```python
from build123d import *

# Parameters (mm, degrees)
BOSS_EXTRUDE1_DEPTH = 0.6


with BuildPart() as part:
    # Sketch1 → Boss-Extrude1 (new body)
    with BuildSketch(Plane(origin=(0, 0, 0), x_dir=(1, 0, 0), z_dir=(0, 1, 0))):
        with BuildLine():
            ThreePointArc((7.5, 10), (0, 12.5), (-7.5, 10))
            Line((-7.5, 10), (-7.5, 0.704545455))
            Line((-7.5, 0.704545455), (7.5, 0.704545455))
            Line((7.5, 0.704545455), (7.5, 10))
        make_face()
        with BuildLine():
            Line((-7.5, 0.704545455), (-7.5, 10))
            ThreePointArc((-7.5, 10), (-5.590169944, -11.180339887), (12.5, 0))
            ThreePointArc((12.5, 0), (11.180339887, 5.590169944), (7.5, 10))
            Line((7.5, 10), (7.5, 0.704545455))
            Line((7.5, 0.704545455), (-7.5, 0.704545455))
        make_face()
        with BuildLine():
            Line((7.5, 24.295454545), (-7.5, 24.295454545))
            Line((-7.5, 24.295454545), (-7.5, 10))
            ThreePointArc((-7.5, 10), (0, 12.5), (7.5, 10))
            Line((7.5, 10), (7.5, 24.295454545))
        make_face()
    extrude(amount=BOSS_EXTRUDE1_DEPTH)


solid = part.part
```
Check sheet for the modelled part. Datum: model origin and axes. Units: mm. Round coordinates to 2 decimals unless told otherwise and drop trailing zeros. Write each loop counter-clockwise with the first axis right and the second up, starting at its lowest first coordinate (ties: lowest second). Pieces come first, ordered by that corner, then holes. Notation, with made-up numbers: (-25, 8) -> (-14, 8) arc R28 ccw to (-14, 30) -> close; hole circle Ø3 at (56.5, -18). An arc over 180 degrees is marked (long way). One line per question, with ' | ' between items. Start each with the question number.
1. Sectioned sample at A-A, the plane y = 0.4. Record the cut outline in (x, z).
2. Scan lines: line 1 along X through (y, z) = (0.5, -13); line 2 along X through (y, z) = (0.45, -9.5); line 3 along Z through (x, y) = (-8.25, 0.3). Record each from-to range of solid material in increasing order. Write a range as from..to.
3. Sectioned sample at B-B, the plane z = 10. Record the cut outline in (x, y).
4. Sectioned sample at C-C, the plane x = 8.75. Record the cut outline in (y, z), then the cut area to 3 significant figures.
Taken from the geometry:
1) outline: (-7.5, -24.3) -> (7.5, -24.3) -> (7.5, -10) arc R12.5 ccw (long way) to (-7.5, -10) -> close
2) line 1: x = -7.5..7.5 | line 2: x = -8.12..8.12 | line 3: z = -9.39..9.39
3) outline: (-7.5, 0) -> (7.5, 0) -> (7.5, 0.6) -> (-7.5, 0.6) -> close
4) outline: (0, -8.93) -> (0.6, -8.93) -> (0.6, 8.93) -> (0, 8.93) -> close | area: 10.7 mm^2
